from build123d import *

# Parameters (mm, degrees)
EXTRUDE_THIN1_DEPTH    = 152.5
CONVERT_SOLID1_START   = -152.5
CONVERT_SOLID1_DEPTH   = 305
CONVERT_SOLID1_2_DEPTH = 305
FILLET1_R              = 2


# Read off the part's stored shape, not the designer's step: Convert-Solid1
with BuildPart() as part:
    # Sketch1 → Extrude-Thin1 (new, symmetric)
    with BuildSketch(Plane.XY):
        Polygon((-50, -60), (-50, 0), (50, 0), (50, -60), (46, -60), (46, -4), (-46, -4), (-46, -60), align=None)
    extrude(amount=EXTRUDE_THIN1_DEPTH, both=True)

    # Convert-Solid1 outline → Convert-Solid1 (cut)
    with BuildSketch(Plane.XY.offset(CONVERT_SOLID1_START)):
        with BuildLine():
            Line((50, 0), (44, 0))
            ThreePointArc((44, 0), (48.242640687, -1.757359313), (50, -6))
            Line((50, -6), (50, 0))
        make_face()
        with BuildLine():
            ThreePointArc((-50, -6), (-48.242640687, -1.757359313), (-44, 0))
            Line((-44, 0), (-50, 0))
            Line((-50, 0), (-50, -6))
        make_face()
    extrude(amount=CONVERT_SOLID1_DEPTH, mode=Mode.SUBTRACT)

    # Convert-Solid1 2 outline → Convert-Solid1 2 (add)
    with BuildSketch(Plane.XY.offset(CONVERT_SOLID1_START)):
        with BuildLine():
            Line((46, -4), (44, -4))
            ThreePointArc((44, -4), (45.414213562, -4.585786438), (46, -6))
            Line((46, -6), (46, -4))
        make_face()
        with BuildLine():
            ThreePointArc((-46, -6), (-45.414213562, -4.585786438), (-44, -4))
            Line((-44, -4), (-46, -4))
            Line((-46, -4), (-46, -6))
        make_face()
    extrude(amount=CONVERT_SOLID1_2_DEPTH)

    # Fillet1
    fillet1_edges = [part.edges().sort_by_distance(p)[0] for p in [
        (48, -60, 152.5),
        (48, -60, -152.5),
        (-48, -60, -152.5),
        (-48, -60, 152.5),
    ]]
    fillet(fillet1_edges, radius=FILLET1_R)


solid = part.part
Input: part model. Units: mm. Frame: model coordinates. A direction names the side the tool comes from. Round coordinates to 2 decimals unless told otherwise and drop trailing zeros. Order: outer loops, then holes, each group sorted by start corner. A loop starts at its lowest first (then second) coordinate and runs counter-clockwise, first axis right, second up. Notation, with made-up numbers: (43.5, 51) - (62.5, 51) arc R9 ccw to (62.5, 58) - close; hole circle Ø6 at (76, -21.75). An arc over 180 degrees is marked (long way). Answer as a JSON object with one key per item and string values. Group by question number.
(1) Cut plane B-B (z = -64). Return loops of the section in (x, y).
(2) Pin query (flat end, axial travel): P1, Ø5, axis at x = -35, z = -79.5, coming from the -Y side. Return the tip coordinate at first contact, or that it passes through.
(3) Cut plane A-A (y = -12.5). Return loops of the section in (x, z), then the cut area to 3 significant figures.
(4) Cut plane C-C (x = -8). Return loops of the section in (y, z).
(5) Draft query along X for faces 1 (the face through (-46, -33, 2)), 2 (the face through (-4, -3, -152.5)), 3 (the face through (1, -4, 2)), 4 (the face through (-48.289, -1.804, -2.135)). Return one class per face: released by +X, released by -X, zero draft, split by the parting line, or undercut.
(6) Reachability of faces 5 (the face through (-1, 0, 2)), 6 (the face through (46, -33, 2)) from +Z, -Z, +X, -X, +Y, -Y: full face, straight path, thin tool, end or side. Return the list, or none.
(7) Material intervals for probe 1 along X at (y, z) = (-23, -65.5); probe 2 along Y at (x, z) = (-2, -133.5); probe 3 along X at (y, z) = (-3.5, -115.5), sorted ascending. Write a range as from..to.
Here are the results:
{
 "1": {"outline": "(-50, -60) - (-46, -60) - (-46, -6) arc R2 cw to (-44, -4) - (44, -4) arc R2 cw to (46, -6) - (46, -60) - (50, -60) - (50, -6) arc R6 ccw to (44, 0) - (-44, 0) arc R6 ccw to (-50, -6) - close"},
 "2": {"P1": "stops at y = -4"},
 "3": {"outline": "(-50, -152.5) - (-46, -152.5) - (-46, 152.5) - (-50, 152.5) - close; (46, -152.5) - (50, -152.5) - (50, 152.5) - (46, 152.5) - close", "area": "2,440 mm^2"},
 "4": {"outline": "(-4, -152.5) - (0, -152.5) - (0, 152.5) - (-4, 152.5) - close"},
 "5": {"face 1": "undercut", "face 2": "zero draft", "face 3": "undercut", "face 4": "released by -X"},
 "6": {"face 5": "+Z, -Z, +X, -X, +Y", "face 6": "+Z, -Z, -Y"},
 "7": {"probe 1": "x = -50..-46, 46..50", "probe 2": "y = -4..0", "probe 3": "x = -49.45..49.45"}
}
